```python
from build123d import *

# Parameters (mm, degrees)
F1_DEPTH = 1
F2_R     = 60.5
F3_DEPTH = 1
F5_DEPTH = 0.2


with BuildPart() as f1:
    # F0 (on Top) → F1 (new body)
    with BuildSketch(Plane.XY):
        with BuildLine():
            Line((-53.027665, 124.93312), (-54.98666, 124.93312))
            ThreePointArc((-54.98666, 124.93312), (-56.400873, 124.347334), (-56.98666, 122.93312))
            Line((-56.98666, 122.93312), (-56.98666, -61.30676))
            ThreePointArc((-56.98666, -61.30676), (-56.400873, -62.720974), (-54.98666, -63.30676))
            Line((-54.98666, -63.30676), (73.152434, -63.30676))
            ThreePointArc((73.152434, -63.30676), (74.566648, -62.720974), (75.152434, -61.30676))
            Line((75.152434, -61.30676), (75.152434, 55.722097))
            ThreePointArc((75.152434, 55.722097), (75.019783, 56.438345), (74.639423, 57.059581))
            Line((74.639423, 57.059581), (72.826351, 59.075319))
            ThreePointArc((72.826351, 59.075319), (72.445992, 59.696556), (72.31334, 60.412804))
            Line((72.31334, 60.412804), (72.31334, 121.015311))
            ThreePointArc((72.31334, 121.015311), (71.727554, 122.429524), (70.31334, 123.015311))
            Line((70.31334, 123.015311), (28.457738, 123.015311))
            Line((28.457738, 123.015311), (28.457738, 124.242901))
            ThreePointArc((28.457738, 124.242901), (28.308866, 125.000085), (27.884411, 125.644545))
            Line((27.884411, 125.644545), (26.658998, 126.89184))
            ThreePointArc((26.658998, 126.89184), (26.00586, 127.334551), (25.232325, 127.490196))
            Line((25.232325, 127.490196), (23.160365, 127.490196))
            ThreePointArc((23.160365, 127.490196), (22.59987, 127.410052), (22.084295, 127.176042))
            Line((22.084295, 127.176042), (21.135774, 126.570603))
            ThreePointArc((21.135774, 126.570603), (20.657619, 126.143481), (20.339185, 125.587005))
            Line((20.339185, 125.587005), (19.806307, 124.165993))
            Line((19.806307, 124.165993), (-13.606119, 124.165993))
            Line((-13.606119, 124.165993), (-13.776735, 124.306503))
            ThreePointArc((-13.776735, 124.306503), (-14.372773, 124.645163), (-15.04816, 124.762651))
            Line((-15.04816, 124.762651), (-44.504093, 124.762651))
            Line((-44.504093, 124.762651), (-45.951107, 126.450838))
            ThreePointArc((-45.951107, 126.450838), (-46.633907, 126.966283), (-47.469622, 127.149258))
            Line((-47.469622, 127.149258), (-50.639777, 127.149258))
            ThreePointArc((-50.639777, 127.149258), (-51.665353, 126.866289), (-52.400722, 126.097452))
            Line((-52.400722, 126.097452), (-53.027665, 124.93312))
        make_face()
    extrude(amount=F1_DEPTH)

    # F2 (on face) → F3 (join)
    with BuildSketch(Plane.XY.offset(1)):
        with BuildLine():
            Line((-15.04816, 124.762651), (-44.504093, 124.762651))
            Line((-44.504093, 124.762651), (-45.951107, 126.450838))
            ThreePointArc((-45.951107, 126.450838), (-46.633907, 126.966283), (-47.469622, 127.149258))
            Line((-47.469622, 127.149258), (-50.639777, 127.149258))
            ThreePointArc((-50.639777, 127.149258), (-51.665353, 126.866289), (-52.400722, 126.097452))
            Line((-52.400722, 126.097452), (-53.027665, 124.93312))
            Line((-53.027665, 124.93312), (-54.98666, 124.93312))
            ThreePointArc((-54.98666, 124.93312), (-56.400873, 124.347334), (-56.98666, 122.93312))
            Line((-56.98666, 122.93312), (-56.98666, -61.30676))
            ThreePointArc((-56.98666, -61.30676), (-56.400873, -62.720974), (-54.98666, -63.30676))
            Line((-54.98666, -63.30676), (73.152434, -63.30676))
            ThreePointArc((73.152434, -63.30676), (74.566648, -62.720974), (75.152434, -61.30676))
            Line((75.152434, -61.30676), (75.152434, 55.722097))
            ThreePointArc((75.152434, 55.722097), (75.019783, 56.438345), (74.639423, 57.059581))
            Line((74.639423, 57.059581), (72.826351, 59.075319))
            ThreePointArc((72.826351, 59.075319), (72.445992, 59.696556), (72.31334, 60.412804))
            Line((72.31334, 60.412804), (72.31334, 121.015311))
            ThreePointArc((72.31334, 121.015311), (71.727554, 122.429524), (70.31334, 123.015311))
            Line((70.31334, 123.015311), (28.457738, 123.015311))
            Line((28.457738, 123.015311), (28.457738, 124.242901))
            ThreePointArc((28.457738, 124.242901), (28.308866, 125.000085), (27.884411, 125.644545))
            Line((27.884411, 125.644545), (26.658998, 126.89184))
            ThreePointArc((26.658998, 126.89184), (26.00586, 127.334551), (25.232325, 127.490196))
            Line((25.232325, 127.490196), (23.160365, 127.490196))
            ThreePointArc((23.160365, 127.490196), (22.59987, 127.410052), (22.084295, 127.176042))
            Line((22.084295, 127.176042), (21.135774, 126.570603))
            ThreePointArc((21.135774, 126.570603), (20.657619, 126.143481), (20.339185, 125.587005))
            Line((20.339185, 125.587005), (19.806307, 124.165993))
            Line((19.806307, 124.165993), (-13.606119, 124.165993))
            Line((-13.606119, 124.165993), (-13.776735, 124.306503))
            ThreePointArc((-13.776735, 124.306503), (-14.372773, 124.645163), (-15.04816, 124.762651))
        make_face()
        with Locations((8.348013, 24.711499)):
            Circle(F2_R, mode=Mode.SUBTRACT)
    extrude(amount=F3_DEPTH)

    # F4 (on face) → F5 (cut)
    with BuildSketch(Plane.XY.offset(2)):
        with BuildLine():
            ThreePointArc((-47.045743, -35.636087), (-47.40188, -35.781107), (-47.549743, -36.136071))
            Line((-47.549743, -36.136071), (-47.549743, -37.502152))
            ThreePointArc((-47.549743, -37.502152), (-47.403297, -37.855705), (-47.049743, -38.002152))
            Line((-47.049743, -38.002152), (-45.490037, -38.002152))
            ThreePointArc((-45.490037, -38.002152), (-45.136483, -38.148599), (-44.990037, -38.502152))
            Line((-44.990037, -38.502152), (-44.990037, -47.598776))
            ThreePointArc((-44.990037, -47.598776), (-45.136483, -47.95233), (-45.490037, -48.098776))
            Line((-45.490037, -48.098776), (-47.002343, -48.098776))
            ThreePointArc((-47.002343, -48.098776), (-47.355896, -48.245223), (-47.502343, -48.598776))
            Line((-47.502343, -48.598776), (-47.502343, -49.893432))
            ThreePointArc((-47.502343, -49.893432), (-47.355896, -50.246986), (-47.002343, -50.393432))
            Line((-47.002343, -50.393432), (-36.445047, -50.393432))
            ThreePointArc((-36.445047, -50.393432), (-36.091493, -50.246986), (-35.945047, -49.893432))
            Line((-35.945047, -49.893432), (-35.945047, -36.220909))
            ThreePointArc((-35.945047, -36.220909), (-36.090082, -35.868773), (-36.441047, -35.720925))
            Line((-36.441047, -35.720925), (-47.045743, -35.636087))
        make_face()
        with BuildLine():
            Line((2.716971, -48.799027), (1.096801, -48.799027))
            ThreePointArc((1.096801, -48.799027), (0.739559, -48.949201), (0.596911, -49.309514))
            Line((0.596911, -49.309514), (0.815092, -59.709521))
            ThreePointArc((0.815092, -59.709521), (0.965156, -60.056275), (1.314982, -60.199033))
            Line((1.314982, -60.199033), (15.472221, -60.199033))
            ThreePointArc((15.472221, -60.199033), (15.825775, -60.052587), (15.972221, -59.699033))
            Line((15.972221, -59.699033), (15.972221, -49.299027))
            ThreePointArc((15.972221, -49.299027), (15.825775, -48.945473), (15.472221, -48.799027))
            Line((15.472221, -48.799027), (13.761731, -48.799027))
            ThreePointArc((13.761731, -48.799027), (13.408177, -48.945473), (13.261731, -49.299027))
            Line((13.261731, -49.299027), (13.261731, -50.212314))
            ThreePointArc((13.261731, -50.212314), (13.115284, -50.565867), (12.761731, -50.712314))
            Line((12.761731, -50.712314), (3.716971, -50.712314))
            ThreePointArc((3.716971, -50.712314), (3.363418, -50.565867), (3.216971, -50.212314))
            Line((3.216971, -50.212314), (3.216971, -49.299027))
            ThreePointArc((3.216971, -49.299027), (3.070525, -48.945473), (2.716971, -48.799027))
        make_face()
        with BuildLine():
            ThreePointArc((53.303006, -35.632055), (52.949453, -35.778502), (52.803006, -36.132055))
            Line((52.803006, -36.132055), (52.803006, -49.733994))
            ThreePointArc((52.803006, -49.733994), (52.949453, -50.087547), (53.303006, -50.233994))
            Line((53.303006, -50.233994), (64.16683, -50.233994))
            ThreePointArc((64.16683, -50.233994), (64.520383, -50.087547), (64.66683, -49.733994))
            Line((64.66683, -49.733994), (64.66683, -48.598776))
            ThreePointArc((64.66683, -48.598776), (64.520383, -48.245223), (64.16683, -48.098776))
            Line((64.16683, -48.098776), (62.550562, -48.098776))
            ThreePointArc((62.550562, -48.098776), (62.197009, -47.95233), (62.050562, -47.598776))
            Line((62.050562, -47.598776), (62.050562, -38.696225))
            ThreePointArc((62.050562, -38.696225), (62.197009, -38.342671), (62.550562, -38.196225))
            Line((62.550562, -38.196225), (64.021894, -38.196225))
            ThreePointArc((64.021894, -38.196225), (64.375447, -38.049778), (64.521894, -37.696225))
            Line((64.521894, -37.696225), (64.521894, -36.132055))
            ThreePointArc((64.521894, -36.132055), (64.375447, -35.778502), (64.021894, -35.632055))
            Line((64.021894, -35.632055), (53.303006, -35.632055))
        make_face()
        with BuildLine():
            ThreePointArc((70.248886, 4.685054), (69.731416, 4.718573), (69.462516, 4.275186))
            Line((69.462516, 4.275186), (69.462516, -1.483415))
            ThreePointArc((69.462516, -1.483415), (69.728887, -1.925475), (70.244185, -1.896529))
            Line((70.244185, -1.896529), (74.415556, 0.94759))
            ThreePointArc((74.415556, 0.94759), (74.63388, 1.357847), (74.420258, 1.770572))
            Line((74.420258, 1.770572), (70.248886, 4.685054))
        make_face()
        with BuildLine():
            Line((-53.041739, 5.185619), (-56.952399, 2.209391))
            ThreePointArc((-56.952399, 2.209391), (-57.14958, 1.808048), (-56.946856, 1.409475))
            Line((-56.946856, 1.409475), (-53.036195, -1.482046))
            ThreePointArc((-53.036195, -1.482046), (-52.5138, -1.526457), (-52.238931, -1.080008))
            Line((-52.238931, -1.080008), (-52.238931, 4.78774))
            ThreePointArc((-52.238931, 4.78774), (-52.516899, 5.235738), (-53.041739, 5.185619))
        make_face()
        with BuildLine():
            ThreePointArc((1.466782, 109.224265), (1.114987, 109.076864), (0.969499, 108.724273))
            Line((0.969499, 108.724273), (0.969499, 98.56072))
            ThreePointArc((0.969499, 98.56072), (1.115946, 98.207166), (1.469499, 98.06072))
            Line((1.469499, 98.06072), (2.701668, 98.06072))
            ThreePointArc((2.701668, 98.06072), (3.055221, 98.207166), (3.201668, 98.56072))
            Line((3.201668, 98.56072), (3.201668, 99.234843))
            ThreePointArc((3.201668, 99.234843), (3.348114, 99.588396), (3.701668, 99.734843))
            Line((3.701668, 99.734843), (12.666707, 99.734843))
            ThreePointArc((12.666707, 99.734843), (13.02026, 99.588396), (13.166707, 99.234843))
            Line((13.166707, 99.234843), (13.166707, 98.401277))
            ThreePointArc((13.166707, 98.401277), (13.313154, 98.047724), (13.666707, 97.901277))
            Line((13.666707, 97.901277), (15.138037, 97.901277))
            ThreePointArc((15.138037, 97.901277), (15.49159, 98.047724), (15.638037, 98.401277))
            Line((15.638037, 98.401277), (15.638037, 108.798559))
            ThreePointArc((15.638037, 108.798559), (15.490628, 109.153072), (15.135319, 109.298552))
            Line((15.135319, 109.298552), (1.466782, 109.224265))
        make_face()
    extrude(amount=-F5_DEPTH, mode=Mode.SUBTRACT)


solid = f1.part
```
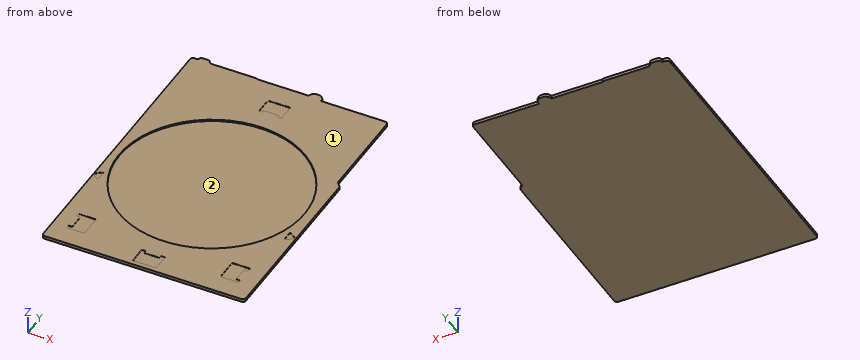
Verification items for the finished model (mm, model axes). Face numbers are marked on the shaded views. Give positions to 0.01 mm unless a question says otherwise; leave off trailing zeros. Order: outer loops, then holes, each group sorted by start corner. A loop starts at its lowest first (then second) coordinate and runs counter-clockwise, first axis right, second up. Notation, with made-up numbers: M 58,-37 L 76,-37 A8 ccw 76,-24 Z; hole C -18,-8.75 d8. An arc over 180 degrees is marked long. Return JSON: item names as keys, results as strings. Group by question number.
1) Section check C-C on x = 33.5. Record the cut outline in (y, z), and give its area (3 significant figures).
2) Section check B-B on y = 22. Record the cut outline in (x, z), and give its area (3 significant figures).
3) Go/stop test with flat-tipped pins: pin 1 Ø1 at (y, z) = (83, 0.5) entering from +X; pin 2 Ø10 at (x, y) = (26, 35) entering from +Z; pin 3 Ø1 at (x, z) = (55.5, 0.5) entering from +Y. Record where each tip stops, or that it passes through.
4) Scan lines: line 1 (Z direction, x = -43, y = 38.5); line 2 (Y direction, x = -31.5, z = 0.9); line 3 (X direction, y = 106.5, z = 0.7). Record each from-to range of solid material in increasing order.
5) Mould release check, pull along X, two halves, no side actions. Record for the marked faces 1 and 2: pulls with the +X half, pulls with the -X half, needs draft (parallel to the pull), parting line crosses it, or undercut.
Answer block:
{
 "1": {"outline": "M -63.31,0 L 123.02,0 L 123.02,2 L 79.74,2 L 79.74,1 L -30.31,1 L -30.31,2 L -63.31,2 Z", "area": "263 mm^2"},
 "2": {"outline": "M -56.99,0 L 75.15,0 L 75.15,2 L 68.79,2 L 68.79,1 L -52.09,1 L -52.09,2 L -56.99,2 Z", "area": "143 mm^2"},
 "3": {"pin 1": "stops at x = 72.31", "pin 2": "stops at z = 1", "pin 3": "stops at y = 123.02"},
 "4": {"line 1": "z = 0 to 1", "line 2": "y = -63.31 to 124.76", "line 3": "x = -56.99 to 72.31"},
 "5": {"face 1": "needs draft", "face 2": "undercut"}
}
